from build123d import *

# Parameters (mm, degrees)
SALIENTE_EXTRUIR1_DEPTH    = 30
CORTAR_EXTRUIR1_DEPTH      = 15
CORTAR_EXTRUIR1_DEPTH_BACK = 41
CROQUIS2_R                 = 1.6
CROQUIS3_R                 = 2.9
CORTAR_EXTRUIR2_DEPTH      = 3.2


with BuildPart() as part:
    # Croquis1 → Saliente-Extruir1 (new body)
    with BuildSketch(Plane.XY):
        Polygon((-21, 0), (-21, 29), (-13, 29), (-13, 3), (13, 3), (13, 29), (21, 29), (21, 0), align=None)
    extrude(amount=SALIENTE_EXTRUIR1_DEPTH)

    # Croquis2 → Cortar-Extruir1 (cut, two sides: drawn at the far end of the back side and taken through both)
    with BuildSketch(Plane.XZ.offset(-CORTAR_EXTRUIR1_DEPTH_BACK)):
        with Locations(Location((-17, 15, 0), (0, 0, 90))):
            Circle(CROQUIS2_R)
        with Locations(Location((17, 15, 0), (0, 0, 90))):
            Circle(CROQUIS2_R)
    extrude(amount=CORTAR_EXTRUIR1_DEPTH + CORTAR_EXTRUIR1_DEPTH_BACK, mode=Mode.SUBTRACT)

    # Croquis3 → Cortar-Extruir2 (cut)
    with BuildSketch(Plane.XZ):
        with Locations(Location((-17, 15, 0), (0, 0, 270))):
            Circle(CROQUIS3_R)
        with Locations(Location((17, 15, 0), (0, 0, 90))):
            Circle(CROQUIS3_R)
    extrude(amount=-CORTAR_EXTRUIR2_DEPTH, mode=Mode.SUBTRACT)


solid = part.part
Geometry check sheet. Reference: the model listing, model coordinates, mm. A direction names the side the tool comes from. Give positions to 0.01 mm unless a question says otherwise; leave off trailing zeros. Order: outer loops, then holes, each group sorted by start corner. A loop starts at its lowest first (then second) coordinate and runs counter-clockwise, first axis right, second up. Notation, with made-up numbers: M 37,50 L 93,50 A22 cw 93,78 Z; hole C -35.75,82.5 d8. An arc over 180 degrees is marked long. Use a Markdown table: item, result.
Item 1: Draft check along X on faces 4 (the cylindrical face through (18.765, 1.578, 12.699)), 5 (the flat face through (-21, 14, 15)), 6 (the flat face through (-15, 29, 15)), 7 (the cylindrical face through (-18.765, 1.578, 17.301)). Enter one of: +X half, -X half, draft (parallel to the pull), parting line (faces both ways), or undercut.
Answers follow:
| item | result |
|---|---|
| face 4 | undercut |
| face 5 | -X half |
| face 6 | draft |
| face 7 | undercut |
Item 2: Tool access check on faces 1 (the flat face through (-13, 16, 15)), 2 (the flat face through (0, 2, 0)), 3 (the flat face through (-18.25, 3.2, 13.75)). Record the directions out of +Z, -Z, +X, -X, +Y, -Y that give a thin tool (end or side, any length) a straight path to the whole face; none if there is none.
Answers follow:
| item | result |
|---|---|
| face 1 | +Z, -Z, +Y |
| face 2 | -Z, +X, -X, +Y, -Y |
| face 3 | -Y |
Item 3: Depth check by flat-ended pin: P1, Ø8, axis at x = -2.5, z = 20, coming from the +Y side; P2, Ø5, axis at x = -17, z = 15, coming from the -Y side. Enter the tip coordinate at first touch or a pass-through.
Answers follow:
| item | result |
|---|---|
| P1 | stops at y = 3 |
| P2 | stops at y = 3.2 |
Item 4: Section check C-C (y = 21). Record the cut outline in (x, z), and give its area (3 significant figures).
Answers follow:
| item | result |
|---|---|
| outline | M -21,0 L -13,0 L -13,30 L -21,30 Z; M 13,0 L 21,0 L 21,30 L 13,30 Z; hole C -17,15 d3.2; hole C 17,15 d3.2 |
| area | 464 mm2 |
Item 5: Section check D-D (z = 20). Record the cut outline in (x, y).
Answers follow:
| item | result |
|---|---|
| outline | M -21,0 L 21,0 L 21,29 L 13,29 L 13,3 L -13,3 L -13,29 L -21,29 Z |
Item 6: Material ranges on line 1 along X through (y, z) = (1.4, 15); line 2 along X through (y, z) = (21, 15); line 3 along X through (y, z) = (27, 11), recorded low to high.
Answers follow:
| item | result |
|---|---|
| line 1 | x = -21 to -19.9, -14.1 to 14.1, 19.9 to 21 |
| line 2 | x = -21 to -18.6, -15.4 to -13, 13 to 15.4, 18.6 to 21 |
| line 3 | x = -21 to -13, 13 to 21 |
Item 7: Section check B-B (x = 17). Record the cut outline in (y, z).
Answers follow:
| item | result |
|---|---|
| outline | M 0,0 L 29,0 L 29,13.4 L 3.2,13.4 L 3.2,12.1 L 0,12.1 Z; M 0,17.9 L 3.2,17.9 L 3.2,16.6 L 29,16.6 L 29,30 L 0,30 Z |
Item 8: Section check A-A (z = 15). Record the cut outline in (x, y).
Answers follow:
| item | result |
|---|---|
| outline | M -21,0 L -19.9,0 L -19.9,3.2 L -18.6,3.2 L -18.6,29 L -21,29 Z; M -15.4,3.2 L -14.1,3.2 L -14.1,0 L 14.1,0 L 14.1,3.2 L 15.4,3.2 L 15.4,29 L 13,29 L 13,3 L -13,3 L -13,29 L -15.4,29 Z; M 18.6,3.2 L 19.9,3.2 L 19.9,0 L 21,0 L 21,29 L 18.6,29 Z |
